Part model, mm, in its own coordinate system. A direction names the side the tool comes from. Give positions to 0.01 mm unless a question says otherwise; leave off trailing zeros. Write each loop counter-clockwise with the first axis right and the second up, starting at its lowest first coordinate (ties: lowest second). Pieces come first, ordered by that corner, then holes. Notation, with made-up numbers: M 48,-5 L 60,-5 A10 ccw 60,8 Z; hole C 62.25,-35 d3. An arc over 180 degrees is marked long. Use a Markdown table: item, result. Add a question column.
from build123d import *

# Parameters (mm, degrees)
SKETCH3_W                    = 114
SKETCH3_H                    = 40
BASE_FLANGE1_DEPTH           = 3
EDGE_FLANGE1_STRIP_W         = 13.4732
EDGE_FLANGE1_STRIP_H         = 3
EDGE_FLANGE1_STRIP_CUT_DEPTH = 40
EDGE_FLANGE1_DEPTH           = 40
EDGE_FLANGE2_STRIP_W         = 13.4732
EDGE_FLANGE2_STRIP_H         = 3
EDGE_FLANGE2_STRIP_CUT_DEPTH = 40
EDGE_FLANGE2_DEPTH           = 40
SKETCH11_R                   = 8
SKETCH11_R_2                 = 2
CUT_EXTRUDE1_DEPTH           = 10
CUT_EXTRUDE2_REACH           = 157.592
SKETCH12_R                   = 2
CUT_EXTRUDE3_DEPTH           = 156.592416268
CUT_EXTRUDE3_DEPTH_BACK      = 156.592416268
CUT_EXTRUDE4_DEPTH           = 10
FILLET1_R                    = 1


# Sheet-metal steps are written as plain solids
with BuildPart() as part:
    # Sketch3 → Base-Flange1 (new body)
    with BuildSketch(Plane(origin=(0, 0, 0), x_dir=(1, 0, 0), z_dir=(0, 1, 0))):
        Rectangle(SKETCH3_W, SKETCH3_H)
    extrude(amount=-BASE_FLANGE1_DEPTH)

    # Edge-Flange1 strip (across the edge) → Edge-Flange1 strip cut (cut)
    with BuildSketch(Plane(origin=(-57, 0, -20), x_dir=(1, 0, 0), z_dir=(0, 0, 1))):
        with Locations((-6, -1.5)):
            Rectangle(EDGE_FLANGE1_STRIP_W, EDGE_FLANGE1_STRIP_H)
    extrude(amount=EDGE_FLANGE1_STRIP_CUT_DEPTH, mode=Mode.SUBTRACT)

    # Edge-Flange1 section (across the edge) → Edge-Flange1 (add)
    with BuildSketch(Plane(origin=(-57, 0, -20), x_dir=(1, 0, 0), z_dir=(0, 0, 1))):
        with BuildLine():
            Line((-3, 0.7366), (-3, 97))
            Line((-3, 97), (0, 97))
            Line((0, 97), (0, 0.7366))
            ThreePointArc((0, 0.7366), (0.215745145, 0.215745145), (0.7366, 0))
            Line((0.7366, 0), (0.7366, -3))
            ThreePointArc((0.7366, -3), (-1.905575199, -1.905575199), (-3, 0.7366))
        make_face()
    extrude(amount=EDGE_FLANGE1_DEPTH)

    # Edge-Flange2 strip (across the edge) → Edge-Flange2 strip cut (cut)
    with BuildSketch(Plane(origin=(57, 0, 20), x_dir=(-1, 0, 0), z_dir=(0, 0, -1))):
        with Locations((-6, -1.5)):
            Rectangle(EDGE_FLANGE2_STRIP_W, EDGE_FLANGE2_STRIP_H)
    extrude(amount=EDGE_FLANGE2_STRIP_CUT_DEPTH, mode=Mode.SUBTRACT)

    # Edge-Flange2 section (across the edge) → Edge-Flange2 (add)
    with BuildSketch(Plane(origin=(57, 0, 20), x_dir=(-1, 0, 0), z_dir=(0, 0, -1))):
        with BuildLine():
            Line((-3, 0.7366), (-3, 97))
            Line((-3, 97), (0, 97))
            Line((0, 97), (0, 0.7366))
            ThreePointArc((0, 0.7366), (0.215745145, 0.215745145), (0.7366, 0))
            Line((0.7366, 0), (0.7366, -3))
            ThreePointArc((0.7366, -3), (-1.905575199, -1.905575199), (-3, 0.7366))
        make_face()
    extrude(amount=EDGE_FLANGE2_DEPTH)

    # Sketch11 → Cut-Extrude1 (cut)
    with BuildSketch(Plane(origin=(0, -3, 0), x_dir=(-1, 0, 0), z_dir=(0, -1, 0))):
        with Locations(Location((0, 0, 0), (0, 0, 90))):
            Circle(SKETCH11_R)
        with Locations(Location((0, 14, 0), (0, 0, 90))):
            Circle(SKETCH11_R_2)
        with Locations(Location((14, 0, 0), (0, 0, 90))):
            Circle(SKETCH11_R_2)
        with Locations(Location((0, -14, 0), (0, 0, 90))):
            Circle(SKETCH11_R_2)
        with Locations(Location((-14, 0, 0), (0, 0, 90))):
            Circle(SKETCH11_R_2)
        with Locations(Location((50.2634, 6.666666667, 0), (0, 0, 90))):
            Circle(SKETCH11_R_2)
        with Locations(Location((-50.2634, 6.666666667, 0), (0, 0, 90))):
            Circle(SKETCH11_R_2)
        with Locations(Location((50.2634, -6.666666667, 0), (0, 0, 90))):
            Circle(SKETCH11_R_2)
        with Locations(Location((-50.2634, -6.666666667, 0), (0, 0, 90))):
            Circle(SKETCH11_R_2)
    extrude(amount=-CUT_EXTRUDE1_DEPTH, mode=Mode.SUBTRACT)

    # Cut-Extrude2: up to this face of the body (flat: up to its plane)
    cut_extrude2_end = Plane(part.part.faces().sort_by_distance((-60, 48.8683, 0))[0])
    # Sketch12 → Cut-Extrude2 (cut, up to the picked face)
    with BuildSketch(Plane(origin=(60, 0, 0), x_dir=(0, 0, -1), z_dir=(1, 0, 0)), mode=Mode.PRIVATE) as cut_extrude2_sk1:
        with Locations(Location((12.5, 79.674243403, 0), (0, 0, 90))):
            Circle(SKETCH12_R)
    cut_extrude2_tool1 = split(extrude(cut_extrude2_sk1.sketch, amount=-CUT_EXTRUDE2_REACH, mode=Mode.PRIVATE), bisect_by=cut_extrude2_end, keep=Keep.BOTH, mode=Mode.PRIVATE)
    # Sketch12 → Cut-Extrude2 (cut, up to the picked face)
    with BuildSketch(Plane(origin=(60, 0, 0), x_dir=(0, 0, -1), z_dir=(1, 0, 0)), mode=Mode.PRIVATE) as cut_extrude2_sk2:
        with Locations(Location((12.5, 90.674243403, 0), (0, 0, 90))):
            Circle(SKETCH12_R)
    cut_extrude2_tool2 = split(extrude(cut_extrude2_sk2.sketch, amount=-CUT_EXTRUDE2_REACH, mode=Mode.PRIVATE), bisect_by=cut_extrude2_end, keep=Keep.BOTH, mode=Mode.PRIVATE)
    # Sketch12 → Cut-Extrude2 (cut, up to the picked face)
    with BuildSketch(Plane(origin=(60, 0, 0), x_dir=(0, 0, -1), z_dir=(1, 0, 0)), mode=Mode.PRIVATE) as cut_extrude2_sk3:
        with Locations(Location((-12.5, 79.674243403, 0), (0, 0, 90))):
            Circle(SKETCH12_R)
    cut_extrude2_tool3 = split(extrude(cut_extrude2_sk3.sketch, amount=-CUT_EXTRUDE2_REACH, mode=Mode.PRIVATE), bisect_by=cut_extrude2_end, keep=Keep.BOTH, mode=Mode.PRIVATE)
    # Sketch12 → Cut-Extrude2 (cut, up to the picked face)
    with BuildSketch(Plane(origin=(60, 0, 0), x_dir=(0, 0, -1), z_dir=(1, 0, 0)), mode=Mode.PRIVATE) as cut_extrude2_sk4:
        with Locations(Location((-12.5, 90.674243403, 0), (0, 0, 90))):
            Circle(SKETCH12_R)
    cut_extrude2_tool4 = split(extrude(cut_extrude2_sk4.sketch, amount=-CUT_EXTRUDE2_REACH, mode=Mode.PRIVATE), bisect_by=cut_extrude2_end, keep=Keep.BOTH, mode=Mode.PRIVATE)
    add(cut_extrude2_tool1.solids().sort_by(Axis((60, 79.674243, -12.5), (-1, 0, 0)))[0], mode=Mode.SUBTRACT)
    add(cut_extrude2_tool2.solids().sort_by(Axis((60, 90.674243, -12.5), (-1, 0, 0)))[0], mode=Mode.SUBTRACT)
    add(cut_extrude2_tool3.solids().sort_by(Axis((60, 79.674243, 12.5), (-1, 0, 0)))[0], mode=Mode.SUBTRACT)
    add(cut_extrude2_tool4.solids().sort_by(Axis((60, 90.674243, 12.5), (-1, 0, 0)))[0], mode=Mode.SUBTRACT)

    # Sketch14 → Cut-Extrude3 (cut, two sides: drawn at the far end of the back side and taken through both)
    with BuildSketch(Plane(origin=(60, 0, 0), x_dir=(0, 0, -1), z_dir=(1, 0, 0)).offset(-CUT_EXTRUDE3_DEPTH_BACK)):
        Polygon((-12.5, 60.805943605), (-1.641411821, 36.3683), (-12.5, 11.930656395), align=None)
        Polygon((-10.858588179, 64.5), (0, 40.062356395), (10.858588179, 64.5), align=None)
        Polygon((12.5, 60.805943605), (1.641411821, 36.3683), (12.5, 11.930656395), align=None)
        Polygon((10.858588179, 8.2366), (0, 32.674243605), (-10.858588179, 8.2366), align=None)
    extrude(amount=CUT_EXTRUDE3_DEPTH + CUT_EXTRUDE3_DEPTH_BACK, mode=Mode.SUBTRACT)

    # Sketch15 → Cut-Extrude4 (cut)
    with BuildSketch(Plane.XZ.offset(3)):
        Polygon((21, 12.878679656), (33.878679656, 0), (21, -12.878679656), align=None)
        Polygon((23.121320344, 15), (36, 2.121320344), (48.878679656, 15), align=None)
        Polygon((44.2634, 6.142079656), (38.121320344, 0), (44.2634, -6.142079656), align=None)
        Polygon((48.878679656, -15), (36, -2.121320344), (23.121320344, -15), align=None)
        Polygon((-23.121320344, -15), (-48.878679656, -15), (-36, -2.121320344), align=None)
        Polygon((-44.2634, -6.142079656), (-44.2634, 6.142079656), (-38.121320344, 0), align=None)
        Polygon((-48.878679656, 15), (-23.121320344, 15), (-36, 2.121320344), align=None)
        Polygon((-21, -12.878679656), (-21, 12.878679656), (-33.878679656, 0), align=None)
    extrude(amount=-CUT_EXTRUDE4_DEPTH, mode=Mode.SUBTRACT)

    # Fillet1
    fillet1_edges = [part.edges().sort_by_distance(p)[0] for p in [
        (58.5, 60.805943605, -12.5),
        (-58.5, 60.805943605, -12.5),
        (58.5, 11.930656395, -12.5),
        (-58.5, 11.930656395, -12.5),
        (58.5, 36.3683, -1.641411821),
        (-58.5, 36.3683, -1.641411821),
        (58.5, 64.5, 10.858588179),
        (-58.5, 64.5, 10.858588179),
        (58.5, 64.5, -10.858588179),
        (-58.5, 64.5, -10.858588179),
        (58.5, 40.062356395, 0),
        (-58.5, 40.062356395, 0),
        (58.5, 8.2366, -10.858588179),
        (-58.5, 8.2366, -10.858588179),
        (58.5, 8.2366, 10.858588179),
        (-58.5, 8.2366, 10.858588179),
        (58.5, 32.674243605, 0),
        (-58.5, 32.674243605, 0),
        (58.5, 11.930656395, 12.5),
        (-58.5, 11.930656395, 12.5),
        (58.5, 60.805943605, 12.5),
        (-58.5, 60.805943605, 12.5),
        (58.5, 36.3683, 1.641411821),
        (-58.5, 36.3683, 1.641411821),
        (-36, -1.5, -2.121320344),
        (-23.121320344, -1.5, -15),
        (-48.878679656, -1.5, -15),
        (48.878679656, -1.5, -15),
        (23.121320344, -1.5, -15),
        (36, -1.5, -2.121320344),
        (23.121320344, -1.5, 15),
        (48.878679656, -1.5, 15),
        (36, -1.5, 2.121320344),
        (44.2634, -1.5, 6.142079656),
        (44.2634, -1.5, -6.142079656),
        (38.121320344, -1.5, 0),
        (-21, -1.5, -12.878679656),
        (-33.878679656, -1.5, 0),
        (-21, -1.5, 12.878679656),
        (-38.121320344, -1.5, 0),
        (-44.2634, -1.5, -6.142079656),
        (-44.2634, -1.5, 6.142079656),
        (-36, -1.5, 2.121320344),
        (-48.878679656, -1.5, 15),
        (-23.121320344, -1.5, 15),
        (21, -1.5, -12.878679656),
        (21, -1.5, 12.878679656),
        (33.878679656, -1.5, 0),
    ]]
    fillet(fillet1_edges, radius=FILLET1_R)


solid = part.part
1. Cut at A-A (x = -14). Write the cut outline in (y, z).
2. Tool access for faces 1 (the flat face through (58.5, 20.3, 5.5)), 2 (the flat face through (-27.87, -1.52, 6.01)), 3 (the cylindrical face through (-58.88, -1.93, -0.28)): list every direction of +Z, -Z, +X, -X, +Y, -Y with a clear straight run to the whole face (end or side of a thin tool).
3. Cut at B-B (x = 0). Write the cut outline in (y, z), then the cut area to 3 significant figures.
4. Flat gauge pins, fed straight in: pin 1 (1.5 mm diameter, centred on x = 6.5, z = 13, fed in from +Y); pin 2 (1.5 mm diameter, centred on y = -1.5, z = -1.5, fed in from -X); pin 3 (12 mm diameter, centred on y = 28.5, z = 5.5, fed in from -X); pin 4 (0.9 mm diameter, centred on x = -58, z = -4.5, fed in from -Y). Where does each tip first touch, or does it go through?
5. Drill centre lines: probe 1 along X at (y, z) = (15, 12); probe 2 along Y at (x, z) = (47, 9.5). Where is each one in solid material? Low to high. Write a range as [from, to].
6. Cut at D-D (y = 22). Give the number of separate pieces and of enclosed holes in the cut face, then the cut area to 3 significant figures.
7. Mould opens along X. For faces 4 (the flat face through (58, 64.5, 0)), 5 (the flat face through (-42.01, -1.52, -8.13)), 6 (the flat face through (-60, 48, -5)) say: released by +X, released by -X, zero draft, split by the parting line, or undercut.
8. Cut at C-C (y = 34). Write the cut outline in (x, z), then the cut area to 3 significant figures.
A:
| question | item | result |
|---|---|---|
| 1 | outline | M -3,-20 L 0,-20 L 0,-2 L -3,-2 Z; M -3,2 L 0,2 L 0,20 L -3,20 Z |
| 2 | face 1 | +X, -X |
| 2 | face 2 | +Y, -Y |
| 2 | face 3 | +Z, -Z, -X, -Y |
| 3 | outline | M -3,-20 L 0,-20 L 0,-16 L -3,-16 Z; M -3,-12 L 0,-12 L 0,-8 L -3,-8 Z; M -3,8 L 0,8 L 0,12 L -3,12 Z; M -3,16 L 0,16 L 0,20 L -3,20 Z |
| 3 | area | 48.0 mm² |
| 4 | pin 1 | stops at y = 0 |
| 4 | pin 2 | stops at x = -59.69 |
| 4 | pin 3 | stops at x = -60 |
| 4 | pin 4 | stops at y = -2.77 |
| 5 | probe 1 | x = [-60, -57], [57, 60] |
| 5 | probe 2 | y = [-3, 0] |
| 6 | separate pieces | 8 |
| 6 | enclosed holes | 0 |
| 6 | area | 129 mm² |
| 7 | face 4 | zero draft |
| 7 | face 5 | undercut |
| 7 | face 6 | released by -X |
| 8 | outline | M -60,-20 L -57,-20 L -57,-12.5 L -60,-12.5 Z; M -60,-2.69 L -57,-2.69 L -57,2.69 L -60,2.69 Z; M -60,12.5 L -57,12.5 L -57,20 L -60,20 Z; M 57,-20 L 60,-20 L 60,-12.5 L 57,-12.5 Z; M 57,-2.69 L 60,-2.69 L 60,2.69 L 57,2.69 Z; M 57,12.5 L 60,12.5 L 60,20 L 57,20 Z |
| 8 | area | 122 mm² |
